Input: part model. Units: mm. Frame: model coordinates. Face numbers are marked on the shaded views. A direction names the side the tool comes from. Coordinates: 2 decimals unless noted, no trailing zeros. Loops run counter-clockwise (first coordinate to the right, second up) from the corner with the lowest first, then second, coordinate; pieces in that order, holes last. Notation, with made-up numbers: (-4, 49.25) - (23, 49.25) arc R19 cw to (23, 81.25) - close; hole circle Ø3 at (-1.5, -3.5). An arc over 180 degrees is marked (long way). Write item = value, one per line. Start each with the question number.
from build123d import *

# Parameters (mm, degrees)
SKETCH_2_W          = 64.445610825
SKETCH_2_H          = 64.602792554
EXTRUDE_2_DEPTH     = 3
SKETCH_3_R          = 1.5
CUT_EXTRUDE_1_DEPTH = 4
EXTRUDE_3_DEPTH     = 3
EXTRUDE_4_DEPTH     = 3
EXTRUDE_6_DEPTH     = 64.602792554
SKETCH_11_R         = 3
SKETCH_11_R_2       = 1.55
SKETCH_11_R_3       = 9
SKETCH_11_R_4       = 1.05
SKETCH_11_R_5       = 4
EXTRUDE_7_DEPTH     = 2
FILLET_1_R          = 1
FILLET_2_R          = 1
FILLET_3_R          = 1
CUT_EXTRUDE_3_DEPTH = 78.212432343
FILLET_5_R          = 1


with BuildPart() as part:
    # 草图2 → 凸台-拉伸2 (new body)
    with BuildSketch(Plane.XY):
        with Locations((0.170214688, -0.018389364)):
            Rectangle(SKETCH_2_W, SKETCH_2_H)
    extrude(amount=EXTRUDE_2_DEPTH)

    # 草图3 → 切除-拉伸1 (cut)
    with BuildSketch(Plane.XY):
        with Locations((24, -18)):
            Circle(SKETCH_3_R)
        with Locations((-24, -18)):
            Circle(SKETCH_3_R)
        with Locations((-24, 18)):
            Circle(SKETCH_3_R)
        with Locations((24, 18)):
            Circle(SKETCH_3_R)
    extrude(amount=CUT_EXTRUDE_1_DEPTH, mode=Mode.SUBTRACT)

    # 草图9 → 凸台-拉伸3 (add)
    with BuildSketch(Plane(origin=(0, 32.283006913, 0), x_dir=(1, 0, 0), z_dir=(0, 1, 0))):
        Polygon((-32.052590724, -3), (32.393020101, -3), (-23.008931723, -25.383841499), align=None)
        Polygon((-20.798622679, -20.176679707), (11.814804037, -7), (-26.12234685, -7), align=None, mode=Mode.SUBTRACT)
    extrude(amount=-EXTRUDE_3_DEPTH)

    # 草图10 → 凸台-拉伸4 (add)
    with BuildSketch(Plane.XZ.offset(32.319785641)):
        Polygon((-23.008931723, 25.383841499), (-32.052590724, 3), (32.393020101, 3), align=None)
        Polygon((11.814804037, 7), (-20.798622679, 20.176679707), (-26.12234685, 7), align=None, mode=Mode.SUBTRACT)
    extrude(amount=-EXTRUDE_4_DEPTH)

    # 草图13 → 凸台-拉伸6 (add)
    with BuildSketch(Plane(origin=(0, 32.283006913, 0), x_dir=(1, 0, 0), z_dir=(0, 1, 0))):
        Polygon((32.393020101, -3), (33.435007656, -2.579009701), (32.393020101, 0), align=None)
    extrude(amount=-EXTRUDE_6_DEPTH)

    # 草图11 → 凸台-拉伸7 (add)
    # profile 1 of 14: a face of its own
    with BuildSketch(Plane(origin=(5.5877033, 0, 13.830050979), x_dir=(0.9271838545667869, 0, -0.37460659341591335), z_dir=(0.37460659341591335, 0, 0.9271838545667869))):
        with BuildLine():
            Line((30.912964894, 13.360290293), (30.034285238, 14.238969949))
            Line((30.034285238, 14.238969949), (30.034285238, 12.481610636))
            Line((30.034285238, 12.481610636), (33.034285238, 12.481610636))
            ThreePointArc((33.034285238, 12.481610636), (31.886234941, 12.709972039), (30.912964894, 13.360290293))
        make_face()
    # profile 2 of 14: a face of its own
    with BuildSketch(Plane(origin=(5.5877033, 0, 13.830050979), x_dir=(0.9271838545667869, 0, -0.37460659341591335), z_dir=(0.37460659341591335, 0, 0.9271838545667869))):
        with Locations((33.034285238, 15.481610636)):
            Circle(SKETCH_11_R)
        with Locations((33.034285238, 15.481610636)):
            Circle(SKETCH_11_R_2, mode=Mode.SUBTRACT)
    # profile 3 of 14: a face of its own
    with BuildSketch(Plane(origin=(5.5877033, 0, 13.830050979), x_dir=(0.9271838545667869, 0, -0.37460659341591335), z_dir=(0.37460659341591335, 0, 0.9271838545667869))):
        with BuildLine():
            Line((30.034285238, 15.481610693), (30.034285238, 14.238969949))
            Line((30.034285238, 14.238969949), (30.912964894, 13.360290293))
            ThreePointArc((30.912964894, 13.360290293), (30.26264663, 14.333560365), (30.034285238, 15.481610693))
        make_face()
    # profile 4 of 14: a face of its own
    with BuildSketch(Plane(origin=(5.5877033, 0, 13.830050979), x_dir=(0.9271838545667869, 0, -0.37460659341591335), z_dir=(0.37460659341591335, 0, 0.9271838545667869))):
        with BuildLine():
            Line((35.155605582, 17.60293098), (30.034285238, 22.724251323))
            Line((30.034285238, 22.724251323), (30.034285238, 15.481610693))
            ThreePointArc((30.034285238, 15.481610693), (31.886234967, 18.253249245), (35.155605582, 17.60293098))
        make_face()
    # profile 5 of 14: a face of its own
    with BuildSketch(Plane(origin=(5.5877033, 0, 13.830050979), x_dir=(0.9271838545667869, 0, -0.37460659341591335), z_dir=(0.37460659341591335, 0, 0.9271838545667869))):
        with Locations((33.034285238, -15.518389364)):
            Circle(SKETCH_11_R)
        with Locations((33.034285238, -15.518389364)):
            Circle(SKETCH_11_R_2, mode=Mode.SUBTRACT)
    # profile 6 of 14: a face of its own
    with BuildSketch(Plane(origin=(5.5877033, 0, 13.830050979), x_dir=(0.9271838545667869, 0, -0.37460659341591335), z_dir=(0.37460659341591335, 0, 0.9271838545667869))):
        with BuildLine():
            Line((30.912964894, -13.39706902), (30.034285238, -14.275748677))
            Line((30.034285238, -14.275748677), (30.034285238, -15.518389325))
            ThreePointArc((30.034285238, -15.518389325), (30.262646648, -14.370339049), (30.912964894, -13.39706902))
        make_face()
    # profile 7 of 14: a face of its own
    with BuildSketch(Plane(origin=(5.5877033, 0, 13.830050979), x_dir=(0.9271838545667869, 0, -0.37460659341591335), z_dir=(0.37460659341591335, 0, 0.9271838545667869))):
        with BuildLine():
            Line((33.034285238, -12.518389364), (30.034285238, -12.518389364))
            Line((30.034285238, -12.518389364), (30.034285238, -14.275748677))
            Line((30.034285238, -14.275748677), (30.912964894, -13.39706902))
            ThreePointArc((30.912964894, -13.39706902), (31.886234941, -12.746750766), (33.034285238, -12.518389364))
        make_face()
    # profile 8 of 14: a face of its own
    with BuildSketch(Plane(origin=(5.5877033, 0, 13.830050979), x_dir=(0.9271838545667869, 0, -0.37460659341591335), z_dir=(0.37460659341591335, 0, 0.9271838545667869))):
        with BuildLine():
            ThreePointArc((35.155605582, -17.639709707), (31.886234923, -18.290027954), (30.034285238, -15.518389325))
            Line((30.034285238, -15.518389325), (30.034285238, -22.761030051))
            Line((30.034285238, -22.761030051), (35.155605582, -17.639709707))
        make_face()
    # profile 9 of 14: a face of its own
    with BuildSketch(Plane(origin=(5.5877033, 0, 13.830050979), x_dir=(0.9271838545667869, 0, -0.37460659341591335), z_dir=(0.37460659341591335, 0, 0.9271838545667869))):
        with BuildLine():
            Line((20.475529648, -32.319785641), (11.990248274, -32.319785641))
            Line((11.990248274, -32.319785641), (-1.337035106, -45.64706902))
            ThreePointArc((-1.337035106, -45.64706902), (1.148246269, -47.404428333), (2.905605582, -49.889709707))
            Line((2.905605582, -49.889709707), (20.475529648, -32.319785641))
        make_face()
    # profile 10 of 14: a face of its own
    with BuildSketch(Plane(origin=(5.5877033, 0, 13.830050979), x_dir=(0.9271838545667869, 0, -0.37460659341591335), z_dir=(0.37460659341591335, 0, 0.9271838545667869))):
        with Locations((-5.215714762, -53.768389364)):
            Circle(SKETCH_11_R_3)
        with Locations((-11.215714762, -53.768389364)):
            Circle(SKETCH_11_R_4, mode=Mode.SUBTRACT)
        with Locations((-5.215714762, -53.768389364)):
            Circle(SKETCH_11_R_5, mode=Mode.SUBTRACT)
        with Locations((-5.215714762, -47.768389364)):
            Circle(SKETCH_11_R_4, mode=Mode.SUBTRACT)
        with Locations((0.784285238, -53.768389364)):
            Circle(SKETCH_11_R_4, mode=Mode.SUBTRACT)
        with Locations((-5.215714762, -59.768389364)):
            Circle(SKETCH_11_R_4, mode=Mode.SUBTRACT)
    # profile 11 of 14: a face of its own
    with BuildSketch(Plane(origin=(5.5877033, 0, 13.830050979), x_dir=(0.9271838545667869, 0, -0.37460659341591335), z_dir=(0.37460659341591335, 0, 0.9271838545667869))):
        with BuildLine():
            Line((-10.430004789, -46.432778993), (-24.542998142, -32.319785641))
            Line((-24.542998142, -32.319785641), (-28.785638829, -32.319785641))
            Line((-28.785638829, -32.319785641), (-12.551325133, -48.554099337))
            ThreePointArc((-12.551325133, -48.554099337), (-11.579675793, -47.404428333), (-10.430004789, -46.432778993))
        make_face()
    # profile 12 of 14: a face of its own
    with BuildSketch(Plane(origin=(5.5877033, 0, 13.830050979), x_dir=(0.9271838545667869, 0, -0.37460659341591335), z_dir=(0.37460659341591335, 0, 0.9271838545667869))):
        with BuildLine():
            Line((20.475529648, 32.283006913), (2.905605582, 49.85293098))
            ThreePointArc((2.905605582, 49.85293098), (1.148246269, 47.367649606), (-1.337035106, 45.610290293))
            Line((-1.337035106, 45.610290293), (11.990248274, 32.283006913))
            Line((11.990248274, 32.283006913), (20.475529648, 32.283006913))
        make_face()
    # profile 13 of 14: a face of its own
    with BuildSketch(Plane(origin=(5.5877033, 0, 13.830050979), x_dir=(0.9271838545667869, 0, -0.37460659341591335), z_dir=(0.37460659341591335, 0, 0.9271838545667869))):
        with BuildLine():
            ThreePointArc((-10.430004789, 46.396000265), (-11.579675793, 47.367649606), (-12.551325133, 48.517320609))
            Line((-12.551325133, 48.517320609), (-28.785638829, 32.283006913))
            Line((-28.785638829, 32.283006913), (-24.542998142, 32.283006913))
            Line((-24.542998142, 32.283006913), (-10.430004789, 46.396000265))
        make_face()
    # profile 14 of 14: a face of its own
    with BuildSketch(Plane(origin=(5.5877033, 0, 13.830050979), x_dir=(0.9271838545667869, 0, -0.37460659341591335), z_dir=(0.37460659341591335, 0, 0.9271838545667869))):
        with Locations((-5.215714762, 53.731610636)):
            Circle(SKETCH_11_R_3)
        with Locations((-11.215714762, 53.731610636)):
            Circle(SKETCH_11_R_4, mode=Mode.SUBTRACT)
        with Locations((-5.215714762, 53.731610636)):
            Circle(SKETCH_11_R_5, mode=Mode.SUBTRACT)
        with Locations((-5.215714762, 59.731610636)):
            Circle(SKETCH_11_R_4, mode=Mode.SUBTRACT)
        with Locations((0.784285238, 53.731610636)):
            Circle(SKETCH_11_R_4, mode=Mode.SUBTRACT)
        with Locations((-5.215714762, 47.731610636)):
            Circle(SKETCH_11_R_4, mode=Mode.SUBTRACT)
    extrude(amount=-EXTRUDE_7_DEPTH)

    # 圆角1
    fillet_1_edges = [part.edges().sort_by_distance(p)[0] for p in [
        (32.393020101, -0.018389364, 0),
    ]]
    fillet(fillet_1_edges, radius=FILLET_1_R)

    # 圆角2
    fillet_2_edges = [part.edges().sort_by_distance(p)[0] for p in [
        (16.330261319, -32.319785641, 8.411241064),
        (24.19767721, -32.319785641, 5.232598715),
        (-21.476482859, -32.319785641, 23.686157226),
        (-17.542774913, -32.319785641, 22.096836051),
        (19.889362671, -32.319785641, 5.894736035),
        (-19.884235479, -32.319785641, 21.964312784),
        (24.19767721, 32.283006913, 5.232598715),
        (16.330261319, 32.283006913, 8.411241064),
        (-17.542774913, 32.283006913, 22.096836051),
        (-21.476482859, 32.283006913, 23.686157226),
        (19.889362671, 32.283006913, 5.894736035),
        (-19.884235479, 32.283006913, 21.964312784),
    ]]
    fillet(fillet_2_edges, radius=FILLET_2_R)

    # 圆角3
    fillet_3_edges = [part.edges().sort_by_distance(p)[0] for p in [
        (-26.12234685, 30.783006913, 7),
        (11.814804037, 30.783006913, 7),
        (-20.798622679, 30.783006913, 20.176679707),
        (-26.12234685, -30.819785641, 7),
        (-20.798622679, -30.819785641, 20.176679707),
        (11.814804037, -30.819785641, 7),
    ]]
    fillet(fillet_3_edges, radius=FILLET_3_R)

    # 草图15 → 切除-拉伸3 (cut, through all)
    with BuildSketch(Plane.XY.offset(3)):
        Polygon((-18, 16), (18, 16), (0, 2.5), align=None)
        Polygon((-22, 14), (-3.333333333, 0), (-22, -14), align=None)
        Polygon((-18, -16), (18, -16), (0, -2.5), align=None)
        Polygon((22, 14), (3.333333333, 0), (22, -14), align=None)
    extrude(amount=-CUT_EXTRUDE_3_DEPTH, mode=Mode.SUBTRACT)

    # 圆角5
    fillet_5_edges = [part.edges().sort_by_distance(p)[0] for p in [
        (-18, -16, 1.5),
        (0, -2.5, 1.5),
        (18, -16, 1.5),
        (-22, -14, 1.5),
        (-22, 14, 1.5),
        (-3.333333333, 0, 1.5),
        (22, 14, 1.5),
        (22, -14, 1.5),
        (3.333333333, 0, 1.5),
        (0, 2.5, 1.5),
        (-18, 16, 1.5),
        (18, 16, 1.5),
    ]]
    fillet(fillet_5_edges, radius=FILLET_5_R)


solid = part.part
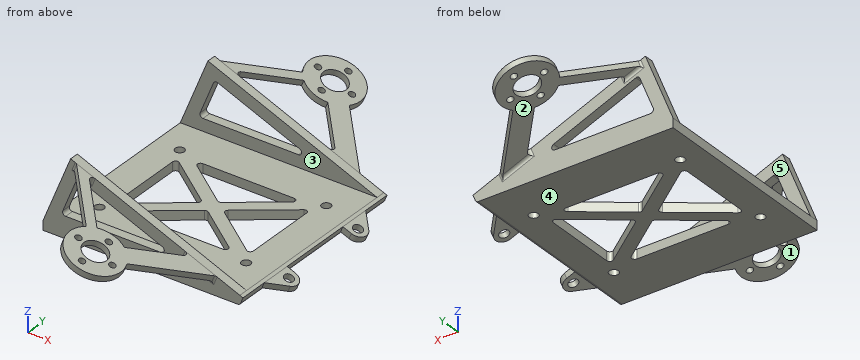
Item 1: Cut plane C-C on y = 25. Return loops of the section in (x, z) (3 decimals), plus the area to 3 significant figures.
Item 2: Cut plane A-A on y = 43.5. Return loops of the section in (x, z), plus the area to 3 significant figures.
Item 3: Access query for the marked faces 1, 2 and 3. Directions: +Z, -Z, +X, -X, +Y, -Y. A direction counts if a zero-diameter tool reaches every point of the face in a straight line with its end or side. Return the directions, or none.
Item 4: Cut plane D-D on y = -21. Return loops of the section in (x, z) (3 decimals), plus the area to 3 significant figures.
Item 5: Ray query, line 1 (Y direction, x = -6, z = 15.25); line 2 (Y direction, x = 24, z = 1.2); line 3 (X direction, y = -18, z = 0.95). Return the intervals inside material, ascending.
Item 6: Pull-direction query (Y, two-part tool) for the marked faces 4 and 5; classes: pulls with the +Y half, pulls with the -Y half, needs draft (parallel to the pull), parting line crosses it, or undercut.
Item 7: Pin query (flat end, axial travel): pin 1 (3.5 mm diameter, centred on x = -16, y = 30.5, fed in from +Z); pin 2 (1.5 mm diameter, centred on y = -1.5, z = 1.5, fed in from +X); pin 3 (2.5 mm diameter, centred on x = 34, z = 1, fed in from +Y); pin 4 (10 mm diameter, centred on x = -23, y = -34, fed in from +Z). Return the tip coordinate at first contact, or that it passes through.
Item 8: Cut plane B-B on x = 27. Return loops of the section in (y, z), plus the area to 3 significant figures.
Recorded:
q1.outline = (-32.053, 0) - (31.719, 0) arc R1 ccw to (32.646, 0.625) - (33.435, 2.579) - (32.393, 3) - (-32.053, 3) - close
q1.area = 195 mm²
q2.outline = (-11.45, 18.56) - (-7.52, 16.97) - (-6.77, 18.82) - (-10.7, 20.41) - close; (5.56, 11.69) - (13.42, 8.51) - (14.17, 10.36) - (6.3, 13.54) - close
q2.area = 25.5 mm²
q3.face_1 = -Z, -X, -Y
q3.face_2 = -Z, -X, +Y
q3.face_3 = +Z, +X, -X
q4.outline = (-32.053, 0) - (31.719, 0) arc R1 ccw to (32.646, 0.625) - (32.686, 0.725) - (34.319, 0.065) - (35.068, 1.919) - (32.393, 3) - (-32.053, 3) - close
q4.area = 198 mm²
q5.line_1 = -32.32 to -29.32, 29.28 to 32.28
q5.line_2 = -32.32 to -19.5, -16.5 to 16.5, 19.5 to 32.28
q5.line_3 = -32.05 to -25.5, -22.5 to 22.5, 25.5 to 37.47
q6.face_4 = needs draft
q6.face_5 = undercut
q7.pin_1 = 23.26
q7.pin_2 = 33.3
q7.pin_3 = 32.28
q7.pin_4 = 25.38
q8.outline = (-32.32, 0) - (32.28, 0) - (32.28, 5.18) - (29.28, 5.18) - (29.28, 3) - (-29.32, 3) - (-29.32, 5.18) - (-32.32, 5.18) - close
q8.area = 207 mm²
